Geometry: final body of the model. Coordinates: model frame, mm. A direction names the side the tool comes from. Coordinates: 2 decimals unless noted, no trailing zeros. Write each loop counter-clockwise with the first axis right and the second up, starting at its lowest first coordinate (ties: lowest second). Pieces come first, ordered by that corner, then holes.
from build123d import *

# Parameters (mm, degrees)
SKETCH1_R               = 6.5
SKETCH1_R_2             = 5
BOSS_EXTRUDE1_DEPTH     = 23
SKETCH2_W               = 13
SKETCH2_H               = 13
BOSS_EXTRUDE2_DEPTH     = 2
CUT_EXTRUDE1_DEPTH      = 25.768932153
CUT_EXTRUDE1_DEPTH_BACK = 25.768932153
SKETCH4_R               = 2
SKETCH5_R               = 2
BOSS_EXTRUDE5_DEPTH     = 4
CHAMFER2_SIZE           = 3
CHAMFER3_SIZE           = 1


# Some blends are built 0.0001 mm under size
with BuildPart() as part:
    # Sketch1 → Boss-Extrude1 (new body)
    with BuildSketch(Plane(origin=(0, 0, 0), x_dir=(0, 0, -1), z_dir=(1, 0, 0))):
        Circle(SKETCH1_R)
        Circle(SKETCH1_R_2, mode=Mode.SUBTRACT)
    extrude(amount=BOSS_EXTRUDE1_DEPTH)

    # Sketch2 → Boss-Extrude2 (add)
    with BuildSketch(Plane(origin=(0, 0, 0), x_dir=(0, 0, -1), z_dir=(1, 0, 0))):
        Rectangle(SKETCH2_W, SKETCH2_H)
    extrude(amount=-BOSS_EXTRUDE2_DEPTH)

    # Sketch4 → Cut-Extrude1 (cut, two sides: drawn at the far end of the back side and taken through both)
    with BuildSketch(Plane(origin=(0, 0, 0), x_dir=(1, 0, 0), z_dir=(0, 1, 0)).offset(-CUT_EXTRUDE1_DEPTH_BACK)):
        with Locations(Location((8, 0, 0), (0, 0, 270))):
            Circle(SKETCH4_R)
        with Locations(Location((18, 0, 0), (0, 0, 270))):
            Circle(SKETCH4_R)
    extrude(amount=CUT_EXTRUDE1_DEPTH + CUT_EXTRUDE1_DEPTH_BACK, mode=Mode.SUBTRACT)

    # Sketch5 → Boss-Extrude5 (add)
    with BuildSketch(Plane(origin=(0, 7, 0), x_dir=(1, 0, 0), z_dir=(0, 1, 0))):
        with BuildLine():
            Line((-2, 7.5), (-2, -7.5))
            Line((-2, -7.5), (-17, -7.5))
            ThreePointArc((-17, -7.5), (-20.061862178, -6.846531969), (-22.590169944, -5))
            Line((-22.590169944, -5), (-42.590169944, -5))
            ThreePointArc((-42.590169944, -5), (-47.590169944, 0), (-42.590169944, 5))
            Line((-42.590169944, 5), (-22.590169944, 5))
            ThreePointArc((-22.590169944, 5), (-20.061862178, 6.846531969), (-17, 7.5))
            Line((-17, 7.5), (-2, 7.5))
        make_face()
        with Locations(Location((-40.590169944, 0, 0), (0, 0, 270))):
            Circle(SKETCH5_R, mode=Mode.SUBTRACT)
        with Locations(Location((-17, 0, 0), (0, 0, 270))):
            Circle(SKETCH5_R, mode=Mode.SUBTRACT)
        with Locations(Location((-31.590169944, 0, 0), (0, 0, 270))):
            Circle(SKETCH5_R, mode=Mode.SUBTRACT)
    boss_extrude5 = extrude(amount=-BOSS_EXTRUDE5_DEPTH)

    # Mirror2: Boss-Extrude5 across plane
    add(boss_extrude5.mirror(Plane.ZX))

    # Chamfer2
    chamfer2_edges = [part.edges().sort_by_distance(p)[0] for p in [
        (-2, 3, 0),
        (-2, -3, 0),
    ]]
    chamfer(chamfer2_edges, length=CHAMFER2_SIZE - 0.0001)  # a hair under: the kernel refuses the full size

    # Chamfer3
    # the kernel refuses this chamfer: 1 mm, written as the material it takes off along each edge
    with BuildSketch(Plane(origin=(0, 9.071682988, -6.5), x_dir=(-0.9996219169112968, 0, -0.027495876610586494), z_dir=(0, -1, 0))) as chamfer3_piece_1_section:
        Polygon((CHAMFER3_SIZE * 0.999621916911, -CHAMFER3_SIZE * 0.0274958766106), (-CHAMFER3_SIZE * 0.0274958766106, -CHAMFER3_SIZE * 0.999621916911), (0, 0), align=None)
    chamfer3_piece_1 = extrude(amount=9.071682988, mode=Mode.PRIVATE)
    chamfer3_piece_1 = chamfer3_piece_1 - Plane(origin=(-0.352424936, 0, 0), x_dir=(0, 0, -1), z_dir=(-1, 0, 0)) * Cylinder(6.5, 23, mode=Mode.PRIVATE)
    add(chamfer3_piece_1, mode=Mode.SUBTRACT)
    with BuildSketch(Plane(origin=(0, 6.5, 2.6e-08), x_dir=(-0.9996219169112968, 0.027495876610586494, 0), z_dir=(0, 0, -1))) as chamfer3_piece_2_section:
        Polygon((CHAMFER3_SIZE * 0.999621916911, -CHAMFER3_SIZE * 0.0274958766106), (-CHAMFER3_SIZE * 0.0274958766106, -CHAMFER3_SIZE * 0.999621916911), (0, 0), align=None)
    chamfer3_piece_2 = extrude(amount=9.071683014, mode=Mode.PRIVATE)
    chamfer3_piece_2 = chamfer3_piece_2 - Plane(origin=(-0.352424936, 0, 0), x_dir=(0, 0, -1), z_dir=(-1, 0, 0)) * Cylinder(6.5, 23, mode=Mode.PRIVATE)
    add(chamfer3_piece_2, mode=Mode.SUBTRACT)
    with BuildSketch(Plane(origin=(0, 6.5, 9.071682988), x_dir=(-0.9996219169112968, 0.027495876610586494, 0), z_dir=(0, 0, -1))) as chamfer3_piece_3_section:
        Polygon((CHAMFER3_SIZE * 0.999621916911, -CHAMFER3_SIZE * 0.0274958766106), (-CHAMFER3_SIZE * 0.0274958766106, -CHAMFER3_SIZE * 0.999621916911), (0, 0), align=None)
    chamfer3_piece_3 = extrude(amount=9.071682962, mode=Mode.PRIVATE)
    chamfer3_piece_3 = chamfer3_piece_3 - Plane(origin=(-0.352424936, 0, 0), x_dir=(0, 0, -1), z_dir=(-1, 0, 0)) * Cylinder(6.5, 23, mode=Mode.PRIVATE)
    add(chamfer3_piece_3, mode=Mode.SUBTRACT)
    with BuildSketch(Plane(origin=(0, -8e-09, 6.5), x_dir=(-0.9996219169112968, 0, 0.027495876610586494), z_dir=(0, 1, 0))) as chamfer3_piece_4_section:
        Polygon((CHAMFER3_SIZE * 0.999621916911, -CHAMFER3_SIZE * 0.0274958766106), (-CHAMFER3_SIZE * 0.0274958766106, -CHAMFER3_SIZE * 0.999621916911), (0, 0), align=None)
    chamfer3_piece_4 = extrude(amount=9.071682996, mode=Mode.PRIVATE)
    chamfer3_piece_4 = chamfer3_piece_4 - Plane(origin=(-0.352424936, 0, 0), x_dir=(0, 0, -1), z_dir=(-1, 0, 0)) * Cylinder(6.5, 23, mode=Mode.PRIVATE)
    add(chamfer3_piece_4, mode=Mode.SUBTRACT)
    with BuildSketch(Plane(origin=(0, -9.071682988, 6.5), x_dir=(-0.9996219169112968, 0, 0.027495876610586494), z_dir=(0, 1, 0))) as chamfer3_piece_5_section:
        Polygon((CHAMFER3_SIZE * 0.999621916911, -CHAMFER3_SIZE * 0.0274958766106), (-CHAMFER3_SIZE * 0.0274958766106, -CHAMFER3_SIZE * 0.999621916911), (0, 0), align=None)
    chamfer3_piece_5 = extrude(amount=9.07168298, mode=Mode.PRIVATE)
    chamfer3_piece_5 = chamfer3_piece_5 - Plane(origin=(-0.352424936, 0, 0), x_dir=(0, 0, -1), z_dir=(-1, 0, 0)) * Cylinder(6.5, 23, mode=Mode.PRIVATE)
    add(chamfer3_piece_5, mode=Mode.SUBTRACT)
    with BuildSketch(Plane(origin=(0, -6.5, 0), x_dir=(-0.9996219169112968, -0.027495876610586494, 0), z_dir=(0, 0, 1))) as chamfer3_piece_6_section:
        Polygon((CHAMFER3_SIZE * 0.999621916911, -CHAMFER3_SIZE * 0.0274958766106), (-CHAMFER3_SIZE * 0.0274958766106, -CHAMFER3_SIZE * 0.999621916911), (0, 0), align=None)
    chamfer3_piece_6 = extrude(amount=9.071682988, mode=Mode.PRIVATE)
    chamfer3_piece_6 = chamfer3_piece_6 - Plane(origin=(-0.352424936, 0, 0), x_dir=(0, 0, -1), z_dir=(-1, 0, 0)) * Cylinder(6.5, 23, mode=Mode.PRIVATE)
    add(chamfer3_piece_6, mode=Mode.SUBTRACT)
    with BuildSketch(Plane(origin=(0, -6.5, -9.071682988), x_dir=(-0.9996219169112968, -0.027495876610586494, 0), z_dir=(0, 0, 1))) as chamfer3_piece_7_section:
        Polygon((CHAMFER3_SIZE * 0.999621916911, -CHAMFER3_SIZE * 0.0274958766106), (-CHAMFER3_SIZE * 0.0274958766106, -CHAMFER3_SIZE * 0.999621916911), (0, 0), align=None)
    chamfer3_piece_7 = extrude(amount=9.071682988, mode=Mode.PRIVATE)
    chamfer3_piece_7 = chamfer3_piece_7 - Plane(origin=(-0.352424936, 0, 0), x_dir=(0, 0, -1), z_dir=(-1, 0, 0)) * Cylinder(6.5, 23, mode=Mode.PRIVATE)
    add(chamfer3_piece_7, mode=Mode.SUBTRACT)
    with BuildSketch(Plane(origin=(0, 0, -6.5), x_dir=(-0.9996219169112968, 0, -0.027495876610586494), z_dir=(0, -1, 0))) as chamfer3_piece_8_section:
        Polygon((CHAMFER3_SIZE * 0.999621916911, -CHAMFER3_SIZE * 0.0274958766106), (-CHAMFER3_SIZE * 0.0274958766106, -CHAMFER3_SIZE * 0.999621916911), (0, 0), align=None)
    chamfer3_piece_8 = extrude(amount=9.071682988, mode=Mode.PRIVATE)
    chamfer3_piece_8 = chamfer3_piece_8 - Plane(origin=(-0.352424936, 0, 0), x_dir=(0, 0, -1), z_dir=(-1, 0, 0)) * Cylinder(6.5, 23, mode=Mode.PRIVATE)
    add(chamfer3_piece_8, mode=Mode.SUBTRACT)


solid = part.part
Item 1: Section C-C, the plane x = 18. Output: boundary loops of the cut face in (y, z).
Derived:
outline: (-6.18, -2) arc R6.5 ccw to (6.18, -2) - (4.58, -2) arc R5 cw to (-4.58, -2) - close; (-6.18, 2) - (-4.58, 2) arc R5 cw to (4.58, 2) - (6.18, 2) arc R6.5 ccw to start
Item 2: Pin query (flat end, axial travel): pin 1 (3 mm diameter, centred on x = -31.5, y = -6, fed in from -Z); pin 2 (4.5 mm diameter, centred on y = 4.5, z = -2, fed in from +X); pin 3 (5 mm diameter, centred on x = 12, z = -5.5, fed in from +Y); pin 4 (4 mm diameter, centred on x = 0.5, z = -1, fed in from +Y). Return the tip coordinate at first contact, or that it passes through.
Derived:
pin 1: stops at z = -5
pin 2: stops at x = 23
pin 3: stops at y = 5.77
pin 4: stops at y = 6.5
Item 3: Material intervals for probe 1 along X at (y, z) = (-4.8, 0); probe 2 along X at (y, z) = (5.95, 0); probe 3 along Y at (x, z) = (-19.5, 0), sorted ascending.
Derived:
probe 1: x = -47.59 to -42.59, -38.59 to -33.59, -29.59 to -19, -15 to 0
probe 2: x = -47.59 to -42.59, -38.59 to -33.59, -29.59 to -19, -15 to 6, 10 to 16, 20 to 23
probe 3: y = -7 to -3, 3 to 7
Item 4: Pull-direction query (X, two-part tool) for faces 1 (the flat face through (0, -5, -5)), 2 (the cylindrical face through (18.601, 5.532, 1.908)), 3 (the flat face through (-19.4, 7, -0.1)), 4 (the cylindrical face through (-47.59, -5.03, 0.11)); classes: released by +X, released by -X, zero draft, split by the parting line, or undercut.
Derived:
face 1: released by +X
face 2: undercut
face 3: zero draft
face 4: released by -X
Item 5: Section D-D, the plane x = 5. Output: boundary loops of the cut face in (y, z), plus the area to 3 significant figures.
Derived:
outline: circle Ø13 at (0, 0); hole circle Ø10 at (0, 0)
area: 54.2 mm2
Item 6: Section A-A, the plane x = -36.5. Output: boundary loops of the cut face in (y, z), plus the area to 3 significant figures.
Derived:
outline: (-7, -5) - (-3, -5) - (-3, 5) - (-7, 5) - close; (3, -5) - (7, -5) - (7, 5) - (3, 5) - close
area: 80.0 mm2
Item 7: Set-up query: faces 5 (the flat face through (-33, -5, -5)), 6 (the flat face through (-2, -6.8, 0)), 7 (the cylindrical face through (11.339, -1.915, -4.619)). Return all of +Z, -Z, +X, -X, +Y, -Y with unobstructed straight access to the full face (end or side cutting, diameter ignored); none if empty.
Derived:
face 5: -Z, -X, +Y, -Y
face 6: +X, -Y
face 7: +X
Item 8: Section B-B, the plane y = 1. Output: boundary loops of the cut face in (x, z).
Derived:
outline: (-3, -6.5) - (-1, -6.5) - (-0.92, -6.42) - (23, -6.42) - (23, -4.9) - (0, -4.9) - (0, 4.9) - (23, 4.9) - (23, 6.42) - (-0.92, 6.42) - (-1, 6.5) - (-3, 6.5) - close
